Input: dimensioned drawing with shaded views. Units: mm. Origin: part minimum x, y, z. Give positions to 0.01 mm unless a question says otherwise; leave off trailing zeros. Write each loop counter-clockwise with the first axis right and the second up, starting at its lowest first coordinate (ties: lowest second). Pieces come first, ordered by that corner, then holes. Notation, with made-up numbers: (86.25, 87.5) -> (119.25, 87.5) arc R17 cw to (119.25, 105.5) -> close; hole circle Ø2 at (14, 77). An arc over 180 degrees is marked (long way). Answer as a JSON object with one key per item and string values.
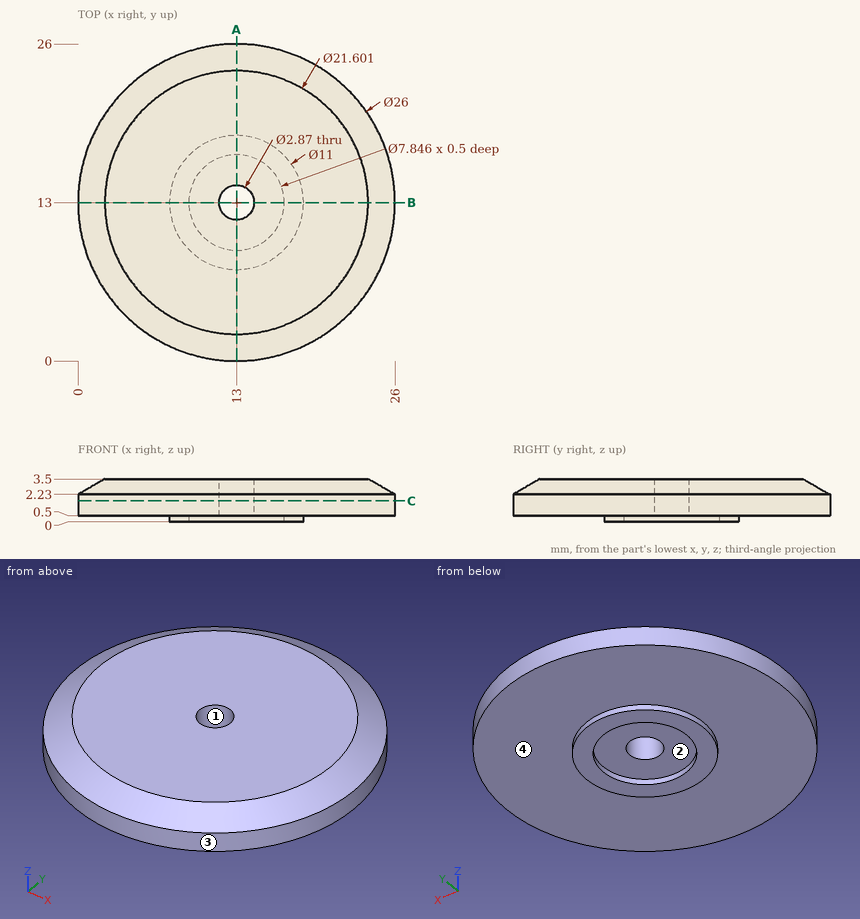
Q1. Cut plane C-C (z = 1.7). Return the cut outline in (x, y) (1 decimal).
Values:
{"outline": "circle Ø26 at (13, 13); hole circle Ø2.9 at (13, 13)"}
Q2. First-contact query: P1, Ø3.5, axis at x = 13, y = 13, coming from the +Z side; P2, Ø4, axis at x = 12, y = 13, coming from the -Z side; P3, Ø1, axis at x = 14.5, z = 1, coming from the +Y side. Flat tips, straight axial feed; report the tip coordinate or a pass-through.
Values:
{"P1": "z = 3.5", "P2": "z = 0.5", "P3": "y = 25.96"}
Q3. Material intervals for L1, parallel to Y at x = 13, z = 0.3; L2, parallel to Y at x = 13, z = 1.1 (1 decimal); L3, parallel to Z at x = 9.75, y = 7, sorted ascending. Write a range as from..to.
Values:
{"L1": "7.5..9.08, 16.92..18.5", "L2": "0..11.6, 14.4..26", "L3": "0.5..3.5"}
Q4. Mould query, pull axis X, two halves, no side actions, for the marked faces 1, 2, 3 and 4. Classes: pulls with the +X half, pulls with the -X half, needs draft (parallel to the pull), parting line crosses it, or undercut.
Values:
{"face 1": "undercut", "face 2": "undercut", "face 3": "parting line crosses it", "face 4": "needs draft"}
Q5. Cut plane A-A (x = 13). Return the cut outline in (y, z) (1 decimal).
Values:
{"outline": "(0, 0.5) -> (7.5, 0.5) -> (7.5, 0) -> (9.1, 0) -> (9.1, 0.5) -> (11.6, 0.5) -> (11.6, 3.5) -> (2.2, 3.5) -> (0, 2.2) -> close; (14.4, 0.5) -> (16.9, 0.5) -> (16.9, 0) -> (18.5, 0) -> (18.5, 0.5) -> (26, 0.5) -> (26, 2.2) -> (23.8, 3.5) -> (14.4, 3.5) -> close"}
